Input: part model. Units: mm. Frame: model coordinates. A direction names the side the tool comes from. Coordinates: 2 decimals unless noted, no trailing zeros. Loops run counter-clockwise (first coordinate to the right, second up) from the corner with the lowest first, then second, coordinate; pieces in that order, holes last. Notation, with made-up numbers: (75, 40.25) -> (103, 40.25) arc R14 ccw to (103, 66.25) -> close; hole circle Ø5 at (33, 5). An arc over 180 degrees is marked (long way). Answer as a JSON object with one key per item and string values.
from build123d import *

# Parameters (mm, degrees)
SKETCH11_R                = 2.6035
F_10_1010_PROFILE_1_DEPTH = 128.27


with BuildPart() as part:
    # Sketch11 → 10 1010 PROFILE(1) (new body)
    with BuildSketch(Plane.ZY):
        with BuildLine():
            Line((-1.709253557, -4.4958), (1.709253557, -4.4958))
            ThreePointArc((1.709253557, -4.4958), (2.922935876, -4.736928798), (3.95226937, -5.423689619))
            Line((3.95226937, -5.423689619), (7.179652728, -8.645192207))
            ThreePointArc((7.179652728, -8.645192207), (7.414733441, -9.822812921), (6.41641086, -10.4902))
            Line((6.41641086, -10.4902), (4.28752, -10.4902))
            ThreePointArc((4.28752, -10.4902), (3.545750844, -10.797450844), (3.2385, -11.53922))
            Line((3.2385, -11.53922), (3.2385, -11.65098))
            ThreePointArc((3.2385, -11.65098), (3.545750844, -12.392749156), (4.28752, -12.7))
            Line((4.28752, -12.7), (5.3171344, -12.7))
            ThreePointArc((5.3171344, -12.7), (5.8251344, -12.192), (6.3331344, -12.7))
            Line((6.3331344, -12.7), (9.5504, -12.7))
            ThreePointArc((9.5504, -12.7), (10.058323491, -12.192000006), (10.566399977, -12.699846982))
            ThreePointArc((10.566399977, -12.699846982), (12.082522516, -12.082522516), (12.699846982, -10.566399977))
            ThreePointArc((12.699846982, -10.566399977), (12.192000006, -10.058323491), (12.7, -9.5504))
            Line((12.7, -9.5504), (12.7, -6.3330836))
            ThreePointArc((12.7, -6.3330836), (12.192, -5.8250836), (12.7, -5.3170836))
            Line((12.7, -5.3170836), (12.7, -4.287470133))
            ThreePointArc((12.7, -4.287470133), (12.392749156, -3.545700977), (11.65098, -3.238450133))
            Line((11.65098, -3.238450133), (11.53922, -3.238450133))
            ThreePointArc((11.53922, -3.238450133), (10.797450844, -3.545700977), (10.4902, -4.287470133))
            Line((10.4902, -4.287470133), (10.4902, -6.402089023))
            ThreePointArc((10.4902, -6.402089023), (9.856394933, -7.351113629), (8.736962546, -7.129240479))
            Line((8.736962546, -7.129240479), (5.440484187, -3.838768792))
            ThreePointArc((5.440484187, -3.838768792), (4.75073678, -2.808015636), (4.5085, -1.591658411))
            Line((4.5085, -1.591658411), (4.5085, 1.591658411))
            ThreePointArc((4.5085, 1.591658411), (4.75073678, 2.808015636), (5.440484187, 3.838768792))
            Line((5.440484187, 3.838768792), (8.736962546, 7.129240479))
            ThreePointArc((8.736962546, 7.129240479), (9.856394933, 7.351113629), (10.4902, 6.402089023))
            Line((10.4902, 6.402089023), (10.4902, 4.287470133))
            ThreePointArc((10.4902, 4.287470133), (10.797450844, 3.545700977), (11.53922, 3.238450133))
            Line((11.53922, 3.238450133), (11.65098, 3.238450133))
            ThreePointArc((11.65098, 3.238450133), (12.392749156, 3.545700977), (12.7, 4.287470133))
            Line((12.7, 4.287470133), (12.7, 5.3171344))
            ThreePointArc((12.7, 5.3171344), (12.192, 5.8251344), (12.7, 6.3331344))
            Line((12.7, 6.3331344), (12.7, 9.5504))
            ThreePointArc((12.7, 9.5504), (12.192000006, 10.058323491), (12.699846982, 10.566399977))
            ThreePointArc((12.699846982, 10.566399977), (12.082522516, 12.082522516), (10.566399977, 12.699846982))
            ThreePointArc((10.566399977, 12.699846982), (10.058323491, 12.192000006), (9.5504, 12.7))
            Line((9.5504, 12.7), (6.3330836, 12.7))
            ThreePointArc((6.3330836, 12.7), (5.8250836, 12.192), (5.3170836, 12.7))
            Line((5.3170836, 12.7), (4.2874692, 12.7))
            ThreePointArc((4.2874692, 12.7), (3.545700044, 12.392749156), (3.2384492, 11.65098))
            Line((3.2384492, 11.65098), (3.2384492, 11.53922))
            ThreePointArc((3.2384492, 11.53922), (3.545700044, 10.797450844), (4.2874692, 10.4902))
            Line((4.2874692, 10.4902), (6.476774195, 10.4902))
            ThreePointArc((6.476774195, 10.4902), (7.43216212, 9.851515102), (7.207191475, 8.724540082))
            Line((7.207191475, 8.724540082), (3.900315394, 5.423689619))
            ThreePointArc((3.900315394, 5.423689619), (2.8709819, 4.736928798), (1.657299581, 4.4958))
            Line((1.657299581, 4.4958), (-1.657299581, 4.4958))
            ThreePointArc((-1.657299581, 4.4958), (-2.8709819, 4.736928798), (-3.900315394, 5.423689619))
            Line((-3.900315394, 5.423689619), (-7.207191475, 8.724540082))
            ThreePointArc((-7.207191475, 8.724540082), (-7.43216212, 9.851515102), (-6.476774195, 10.4902))
            Line((-6.476774195, 10.4902), (-4.2874692, 10.4902))
            ThreePointArc((-4.2874692, 10.4902), (-3.545700044, 10.797450844), (-3.2384492, 11.53922))
            Line((-3.2384492, 11.53922), (-3.2384492, 11.65098))
            ThreePointArc((-3.2384492, 11.65098), (-3.545700044, 12.392749156), (-4.2874692, 12.7))
            Line((-4.2874692, 12.7), (-5.3170836, 12.7))
            ThreePointArc((-5.3170836, 12.7), (-5.8250836, 12.192), (-6.3330836, 12.7))
            Line((-6.3330836, 12.7), (-9.5504, 12.7))
            ThreePointArc((-9.5504, 12.7), (-10.058323491, 12.192000006), (-10.566399977, 12.699846982))
            ThreePointArc((-10.566399977, 12.699846982), (-12.082522516, 12.082522516), (-12.699846982, 10.566399977))
            ThreePointArc((-12.699846982, 10.566399977), (-12.192000006, 10.058323491), (-12.7, 9.5504))
            Line((-12.7, 9.5504), (-12.7, 6.3331344))
            ThreePointArc((-12.7, 6.3331344), (-12.192, 5.8251344), (-12.7, 5.3171344))
            Line((-12.7, 5.3171344), (-12.7, 4.287470133))
            ThreePointArc((-12.7, 4.287470133), (-12.392749156, 3.545700977), (-11.65098, 3.238450133))
            Line((-11.65098, 3.238450133), (-11.53922, 3.238450133))
            ThreePointArc((-11.53922, 3.238450133), (-10.797450844, 3.545700977), (-10.4902, 4.287470133))
            Line((-10.4902, 4.287470133), (-10.4902, 6.402089023))
            ThreePointArc((-10.4902, 6.402089023), (-9.856394933, 7.351113629), (-8.736962546, 7.129240479))
            Line((-8.736962546, 7.129240479), (-5.440484187, 3.838768792))
            ThreePointArc((-5.440484187, 3.838768792), (-4.75073678, 2.808015636), (-4.5085, 1.591658411))
            Line((-4.5085, 1.591658411), (-4.5085, -1.591658411))
            ThreePointArc((-4.5085, -1.591658411), (-4.75073678, -2.808015636), (-5.440484187, -3.838768792))
            Line((-5.440484187, -3.838768792), (-8.736962546, -7.129240479))
            ThreePointArc((-8.736962546, -7.129240479), (-9.856394933, -7.351113629), (-10.4902, -6.402089023))
            Line((-10.4902, -6.402089023), (-10.4902, -4.287470133))
            ThreePointArc((-10.4902, -4.287470133), (-10.797450844, -3.545700977), (-11.53922, -3.238450133))
            Line((-11.53922, -3.238450133), (-11.65098, -3.238450133))
            ThreePointArc((-11.65098, -3.238450133), (-12.392749156, -3.545700977), (-12.7, -4.287470133))
            Line((-12.7, -4.287470133), (-12.7, -5.3170836))
            ThreePointArc((-12.7, -5.3170836), (-12.192, -5.8250836), (-12.7, -6.3330836))
            Line((-12.7, -6.3330836), (-12.7, -9.5504))
            ThreePointArc((-12.7, -9.5504), (-12.192000006, -10.058323491), (-12.699846982, -10.566399977))
            ThreePointArc((-12.699846982, -10.566399977), (-12.082522516, -12.082522516), (-10.566399977, -12.699846982))
            ThreePointArc((-10.566399977, -12.699846982), (-10.058323491, -12.192000006), (-9.5504, -12.7))
            Line((-9.5504, -12.7), (-6.3331344, -12.7))
            ThreePointArc((-6.3331344, -12.7), (-5.8251344, -12.192), (-5.3171344, -12.7))
            Line((-5.3171344, -12.7), (-4.28752, -12.7))
            ThreePointArc((-4.28752, -12.7), (-3.545750844, -12.392749156), (-3.2385, -11.65098))
            Line((-3.2385, -11.65098), (-3.2385, -11.53922))
            ThreePointArc((-3.2385, -11.53922), (-3.545750844, -10.797450844), (-4.28752, -10.4902))
            Line((-4.28752, -10.4902), (-6.41641086, -10.4902))
            ThreePointArc((-6.41641086, -10.4902), (-7.414733441, -9.822812921), (-7.179652728, -8.645192207))
            Line((-7.179652728, -8.645192207), (-3.95226937, -5.423689619))
            ThreePointArc((-3.95226937, -5.423689619), (-2.922935876, -4.736928798), (-1.709253557, -4.4958))
        make_face()
        Circle(SKETCH11_R, mode=Mode.SUBTRACT)
    extrude(amount=F_10_1010_PROFILE_1_DEPTH)


solid = part.part
1. Mould query, pull axis Z, two halves, no side actions, for faces 1 (the face through (-63, 0, 4.508)), 2 (the face through (-63, -12.7, -8)), 3 (the face through (-63.24, 7.05, -5.53)), 4 (the face through (-63, -8, -12.7)). Classes: pulls with the +Z half, pulls with the -Z half, needs draft (parallel to the pull), parting line crosses it, or undercut.
Reply:
{"face 1": "pulls with the +Z half", "face 2": "needs draft", "face 3": "undercut", "face 4": "pulls with the -Z half"}
2. Section query A-A (z = 0). Return loops of the section in (x, y), plus the area to 3 significant figures.
Reply:
{"outline": "(-128.27, -4.5) -> (0, -4.5) -> (0, -2.6) -> (-128.27, -2.6) -> close; (-128.27, 2.6) -> (0, 2.6) -> (0, 4.5) -> (-128.27, 4.5) -> close", "area": "485 mm2"}
3. Pin query (flat end, axial travel): P1, Ø1, axis at x = -62.5, z = 0.5, coming from the -Y side; P2, Ø4, axis at x = -51, y = 0.5, coming from the +Z side; P3, Ø1.6, axis at x = -76, y = 0, coming from the -Z side. Return the tip coordinate at first contact, or that it passes through.
Reply:
{"P1": "stops at y = -4.5", "P2": "stops at z = 4.64", "P3": "stops at z = -4.51"}
4. Line query: line 1 along Z through (x, y) = (-65.5, 3.5); line 2 along Y through (x, z) = (-75, 0); line 3 along Z through (x, y) = (-48.5, -4). Output: solid intervals per line, ascending.
Reply:
{"line 1": "z = -12.34 to -10.85, -5.15 to 5.15, 10.85 to 12.34", "line 2": "y = -4.5 to -2.6, 2.6 to 4.5", "line 3": "z = -12.66 to -10.53, -5.6 to 5.6, 10.53 to 12.66"}
5. Section query B-B (y = 0). Return loops of the section in (x, z).
Reply:
{"outline": "(-128.27, -4.51) -> (0, -4.51) -> (0, -2.6) -> (-128.27, -2.6) -> close; (-128.27, 2.6) -> (0, 2.6) -> (0, 4.51) -> (-128.27, 4.51) -> close"}
6. Access query for faces 5 (the face through (-63.237, -2.824, 4.757)), 6 (the face through (-63, 0, -4.508)), 7 (the face through (-63, 4.496, 0)), 8 (the face through (-63, -4.496, 0)), 9 (the face through (-63, -12.7, 8)). Directions: +Z, -Z, +X, -X, +Y, -Y. A direction counts if a zero-diameter tool reaches every point of the face in a straight line with its end or side. Return the directions, or none.
Reply:
{"face 5": "+X, -X", "face 6": "-Z, +X, -X", "face 7": "+X, -X, +Y", "face 8": "+X, -X, -Y", "face 9": "+Z, -Z, +X, -X, -Y"}
